Input: part model. Units: mm. Frame: model coordinates. A direction names the side the tool comes from. Give positions to 0.01 mm unless a question says otherwise; leave off trailing zeros. Order: outer loops, then holes, each group sorted by start corner. A loop starts at its lowest first (then second) coordinate and runs counter-clockwise, first axis right, second up.
```python
from build123d import *

# Parameters (mm, degrees)
SKETCH_3_W          = 85
SKETCH_3_H          = 21
EXTRUDE_2_DEPTH     = 20
SKETCH_4_R          = 3
CUT_EXTRUDE_2_DEPTH = 49.241579576
CUT_EXTRUDE_3_DEPTH = 49.241579576


with BuildPart() as part:
    # Эскиз3 → Вытянуть2 (new body)
    with BuildSketch(Plane.XY):
        with Locations((0, 0.5)):
            Rectangle(SKETCH_3_W, SKETCH_3_H)
    extrude(amount=EXTRUDE_2_DEPTH)

    # Эскиз4 → Вырез-Вытянуть2 (cut, through all)
    with BuildSketch(Plane.XY.offset(20)):
        with Locations((-34.8, -3.2)):
            Circle(SKETCH_4_R)
        with Locations((34.8, -3.2)):
            Circle(SKETCH_4_R)
    extrude(amount=-CUT_EXTRUDE_2_DEPTH, mode=Mode.SUBTRACT)

    # Эскиз6 → Вырез-Вытянуть3 (cut, through all)
    with BuildSketch(Plane.XY.offset(20)):
        with BuildLine():
            Line((-34.63787593, -10), (34.63787593, -10))
            add(Edge.make_bspline(
                [(25.5, 4.472396239), (29.328176933, 2.427539869), (26.262862424, -9.380662075), (34.63787593, -10)],
                knots=[0, 0, 0, 0, 1, 1, 1, 1], degree=3))
            Line((25.5, 4.472396239), (-25.5, 4.472396239))
            add(Edge.make_bspline(
                [(-25.5, 4.472396239), (-29.328176933, 2.427539869), (-26.262862424, -9.380662075), (-34.63787593, -10)],
                knots=[0, 0, 0, 0, 1, 1, 1, 1], degree=3))
        make_face()
    extrude(amount=-CUT_EXTRUDE_3_DEPTH, mode=Mode.SUBTRACT)


solid = part.part
```
1) Cut plane A-A (z = 4). Count the separate pieces of the cut face and the enclosed holes in it, then the cut area to 3 significant figures.
2) Line query: probe 1 along Y at (x, z) = (-34.8, 8); probe 2 along X at (y, z) = (-4.75, 14); probe 3 along X at (y, z) = (-1.75, 16.25). Output: solid intervals per line, ascending.
3) Pull-direction query (X, two-part tool) for faces 1 (the face through (42.5, 0, 10)), 2 (the face through (39, -10, 10)), 3 (the face through (-37.8, -3.1, 10.1)); classes: pulls with the +X half, pulls with the -X half, needs draft (parallel to the pull), parting line crosses it, or undercut.
4) Cut plane C-C (x = -16.5). Return the cut outline in (y, z), then the cut area to 3 significant figures.
5) Reachability of faces 4 (the face through (37.66, -2.3, 10.14)), 5 (the face through (0, 4.472, 10)) from +Z, -Z, +X, -X, +Y, -Y: full face, straight path, thin tool, end or side. Return the list, or none.
Geometry says:
1. separate pieces: 1
1. enclosed holes: 2
1. area: 901 mm2
2. probe 1: y = -10 to -6.2, -0.2 to 11
2. probe 2: x = -42.5 to -37.37, -32.23 to -28.75, 28.75 to 32.23, 37.37 to 42.5
2. probe 3: x = -42.5 to -37.43, -32.17 to -28.04, 28.04 to 32.17, 37.43 to 42.5
3. face 1: pulls with the +X half
3. face 2: needs draft
3. face 3: undercut
4. outline: (4.47, 0) - (11, 0) - (11, 20) - (4.47, 20) - close
4. area: 131 mm2
5. face 4: +Z, -Z
5. face 5: +Z, -Z, -Y
